For this review, take the finished solid that the model builds, in its own axes (mm). Give positions to 0.01 mm unless a question says otherwise; leave off trailing zeros. Write each loop counter-clockwise with the first axis right and the second up, starting at its lowest first coordinate (ties: lowest second). Pieces come first, ordered by that corner, then holes. Notation, with made-up numbers: (9, 49.5) -> (67, 49.5) arc R12 ccw to (67, 66.5) -> close; hole circle Ø2 at (-12, 33). An arc over 180 degrees is marked (long way). Return JSON: item names as keys, results as strings.
from build123d import *

# Parameters (mm, degrees)
CYLINDER170_R         = 6.5
CYLINDER170_DEPTH     = 10
ARRAY001_COUNT        = 6
ARRAY001_ANGLE        = 170
CYLINDER012_R         = 2.579687
CYLINDER012_DEPTH     = 19.5
ARRAY_COUNT           = 6
ARRAY_ANGLE           = 208
ARRAY_PLACEMENT_ANGLE = 109
CYLINDER052_R         = 47.75
CYLINDER052_DEPTH     = 3
CYLINDER051_R         = 51.25
CYLINDER051_DEPTH     = 3
CYLINDER164_R         = 2.28
CYLINDER164_DEPTH     = 29
CYLINDER163_R         = 2.58
CYLINDER163_DEPTH     = 29
CYLINDER159_R         = 9
CYLINDER159_DEPTH     = 21
CYLINDER165_R         = 4
CYLINDER165_DEPTH     = 10
CYLINDER166_R         = 4
CYLINDER166_DEPTH     = 10
CYLINDER167_R         = 4
CYLINDER167_DEPTH     = 10
CYLINDER168_R         = 4
CYLINDER168_DEPTH     = 10
CYLINDER005_R         = 51
CYLINDER005_DEPTH     = 20
CYLINDER004_R         = 70.0875
CYLINDER004_DEPTH     = 20
BOX_W                 = 193
BOX_H                 = 248
BOX_DEPTH             = 6.2
FILLET_R              = 80


with BuildPart() as array001:
    # Cylinder170 → Cylinder170 (new body)
    with BuildSketch(Plane(origin=(60, 181, 0), x_dir=(1, 0, 0), z_dir=(0, 0, 1))):
        Circle(CYLINDER170_R)
    extrude(amount=CYLINDER170_DEPTH)

    # Array001: Array001 ×6 about axis
    array001_axis = Axis((0, 176, 0), (0, 0, 1))


with BuildPart() as array001_1:
    add(array001.part)
    for i in range(1, ARRAY001_COUNT):
        add(array001.part.rotate(array001_axis, i * ARRAY001_ANGLE / (ARRAY001_COUNT - 1)))


with BuildPart() as array001_2:
    # Array001 placement: moved
    add(array001_1.part.moved(Location((0, -5, 0))))


with BuildPart() as obj1:
    # Cylinder012 → Cylinder012 (new body)
    with BuildSketch(Plane(origin=(36.025, 58.5, -4), x_dir=(1, 0, 0), z_dir=(0, 0, 1))):
        Circle(CYLINDER012_R)
    extrude(amount=CYLINDER012_DEPTH)

    # Array: obj1 ×6 about axis
    array_axis = Axis((0, 0, 0), (0, 0, 1))


with BuildPart() as obj1_1:
    add(obj1.part)
    for i in range(1, ARRAY_COUNT):
        add(obj1.part.rotate(array_axis, i * ARRAY_ANGLE / (ARRAY_COUNT - 1)))


with BuildPart() as obj1_2:
    # Array placement: moved
    add(obj1_1.part.moved(Location((0, 102, 0))).rotate(Axis((0, 102, 0), (0, 0, 1)), ARRAY_PLACEMENT_ANGLE))


with BuildPart() as flange002:
    # Cylinder052 → Cylinder052 (new body)
    with BuildSketch(Plane(origin=(0, 68, 0), x_dir=(1, 0, 0), z_dir=(0, 0, 1))):
        Circle(CYLINDER052_R)
    extrude(amount=CYLINDER052_DEPTH)


with BuildPart() as centeringringgroove:
    # Cylinder051 → Cylinder051 (new body)
    with BuildSketch(Plane(origin=(0, 68, 0), x_dir=(1, 0, 0), z_dir=(0, 0, 1))):
        Circle(CYLINDER051_R)
    extrude(amount=CYLINDER051_DEPTH)

    # Cut001: cut Flange002
    add(flange002.part, mode=Mode.SUBTRACT)


with BuildPart() as centeringringgroove_1:
    # Cut001 placement: moved
    add(centeringringgroove.part.moved(Location((0, 35, 0))))


with BuildPart() as cylinder016:
    # Cylinder164 → Cylinder164 (new body)
    with BuildSketch(Plane(origin=(15, 33, -9), x_dir=(1, 0, 0), z_dir=(0, 0, 1))):
        Circle(CYLINDER164_R)
    extrude(amount=CYLINDER164_DEPTH)


with BuildPart() as cylinder015:
    # Cylinder163 → Cylinder163 (new body)
    with BuildSketch(Plane(origin=(-14.5, 33.7, -7), x_dir=(1, 0, 0), z_dir=(0, 0, 1))):
        Circle(CYLINDER163_R)
    extrude(amount=CYLINDER163_DEPTH)


with BuildPart() as cylinder011:
    # Cylinder159 → Cylinder159 (new body)
    with BuildSketch(Plane(origin=(0, 67, -4), x_dir=(1, 0, 0), z_dir=(0, 0, 1))):
        Circle(CYLINDER159_R)
    extrude(amount=CYLINDER159_DEPTH)


with BuildPart() as cylinder017:
    # Cylinder165 → Cylinder165 (new body)
    with BuildSketch(Plane(origin=(-87, 173, 0), x_dir=(1, 0, 0), z_dir=(0, 0, 1))):
        Circle(CYLINDER165_R)
    extrude(amount=CYLINDER165_DEPTH)


with BuildPart() as cylinder018:
    # Cylinder166 → Cylinder166 (new body)
    with BuildSketch(Plane(origin=(87, 68, 0), x_dir=(1, 0, 0), z_dir=(0, 0, 1))):
        Circle(CYLINDER166_R)
    extrude(amount=CYLINDER166_DEPTH)


with BuildPart() as cylinder019:
    # Cylinder167 → Cylinder167 (new body)
    with BuildSketch(Plane(origin=(-87, 68, 0), x_dir=(1, 0, 0), z_dir=(0, 0, 1))):
        Circle(CYLINDER167_R)
    extrude(amount=CYLINDER167_DEPTH)


with BuildPart() as cylinder020:
    # Cylinder168 → Cylinder168 (new body)
    with BuildSketch(Plane(origin=(87, 173, 0), x_dir=(1, 0, 0), z_dir=(0, 0, 1))):
        Circle(CYLINDER168_R)
    extrude(amount=CYLINDER168_DEPTH)


with BuildPart() as cylinder005:
    # Cylinder005 → Cylinder005 (new body)
    with BuildSketch(Plane(origin=(0, 74, 0), x_dir=(1, 0, 0), z_dir=(0, 0, 1))):
        Circle(CYLINDER005_R)
    extrude(amount=CYLINDER005_DEPTH)


with BuildPart() as fusion001:
    # Cylinder004 → Cylinder004 (new body)
    with BuildSketch(Plane(origin=(0, 149, 0), x_dir=(1, 0, 0), z_dir=(0, 0, 1))):
        Circle(CYLINDER004_R)
    extrude(amount=CYLINDER004_DEPTH)

    # Common: intersect Cylinder005
    add(cylinder005.part, mode=Mode.INTERSECT)


with BuildPart() as fusion001_1:
    # Common placement: moved
    add(fusion001.part.moved(Location((0, 29, 0))))

    # Fusion: union obj1, CenteringRingGroove, Cylinder016, Cylinder015, Cylinder011, Cylinder017, Cylinder018, Cylinder019, Cylinder020
    add(obj1_2.part)
    add(centeringringgroove_1.part)
    add(cylinder016.part)
    add(cylinder015.part)
    add(cylinder011.part)
    add(cylinder017.part)
    add(cylinder018.part)
    add(cylinder019.part)
    add(cylinder020.part)

    # Fusion001: union Array001
    add(array001_2.part)


with BuildPart() as cut021:
    # Box → Box (new body)
    with BuildSketch(Plane(origin=(-96.5, 0, 0), x_dir=(1, 0, 0), z_dir=(0, 0, 1))):
        with Locations((96.5, 124)):
            Rectangle(BOX_W, BOX_H)
    extrude(amount=BOX_DEPTH)

    # Fillet
    fillet_edges = [cut021.edges().sort_by_distance(p)[0] for p in [
        (-96.5, 0, 3.1),
        (-96.5, 248, 3.1),
        (96.5, 0, 3.1),
        (96.5, 248, 3.1),
    ]]
    fillet(fillet_edges, radius=FILLET_R)

    # Cut021: cut Fusion001
    add(fusion001_1.part, mode=Mode.SUBTRACT)


solid = cut021.part
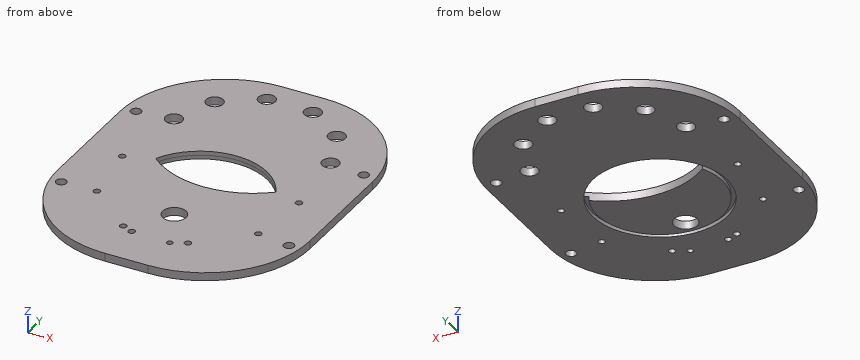
1. Add section A-A, the plane x = 87. State the section outline as (y, z) points, plus the area to 3 significant figures.
Results found:
{"outline": "(42.19, 0) -> (64, 0) -> (64, 6.2) -> (42.19, 6.2) -> close; (72, 0) -> (169, 0) -> (169, 6.2) -> (72, 6.2) -> close; (177, 0) -> (205.81, 0) -> (205.81, 6.2) -> (177, 6.2) -> close", "area": "915 mm²"}
2. Add section D-D, the plane x = -35.5. State the section outline as (y, z) points, plus the area to 3 significant figures.
Results found:
{"outline": "(2.29, 0) -> (66.04, 0) -> (66.04, 3) -> (71.07, 3) -> (71.07, 0) -> (117.57, 0) -> (117.57, 6.2) -> (2.29, 6.2) -> close; (139.62, 3) -> (139.96, 3) -> (139.96, 0) -> (245.71, 0) -> (245.71, 6.2) -> (139.62, 6.2) -> close", "area": "1,360 mm²"}
3. For pin 1 (17 mm diameter, centred on x = 60, y = 176, fed in from -Z); pin 2 (1 mm diameter, centred on x = -32, z = 3, fed in from +Y); pin 3 (1.5 mm diameter, centred on y = 49.5, z = 1.5, fed in from -X), all flat-tipped, find the tip position at first contact; note any pin that passes through.
Results found:
{"pin 1": "stops at z = 0", "pin 2": "stops at y = 246.58", "pin 3": "stops at x = -90.76"}
4. To check wall thickness, follow probe 1 along Y at (x, z) = (-61, 4.5); probe 2 along Y at (x, z) = (87, 3.5); probe 3 along Y at (x, z) = (13, 5). State the ranges of each line that lie inside material, in increasing order.
Results found:
{"probe 1": "y = 13.52 to 66.3, 71.14 to 170.08, 182.91 to 234.48", "probe 2": "y = 42.19 to 64, 72 to 169, 177 to 205.81", "probe 3": "y = 0 to 31.91, 34.09 to 109.13, 152.32 to 224.17, 232.84 to 248"}
5. Add section C-C, the plane y = 103. State the section outline as (x, z) points, plus the area to 3 significant figures.
Results found:
{"outline": "(-96.5, 0) -> (-51.25, 0) -> (-51.25, 3) -> (-47.75, 3) -> (-47.75, 0) -> (47.75, 0) -> (47.75, 3) -> (51.25, 3) -> (51.25, 0) -> (96.5, 0) -> (96.5, 6.2) -> (-96.5, 6.2) -> close", "area": "1,180 mm²"}
6. Add section B-B, the plane y = 143.5. State the section outline as (x, z) points.
Results found:
{"outline": "(-96.5, 0) -> (-31.41, 0) -> (-31.41, 3) -> (-31, 3) -> (-31, 6.2) -> (-96.5, 6.2) -> close; (31, 3) -> (31.41, 3) -> (31.41, 0) -> (96.5, 0) -> (96.5, 6.2) -> (31, 6.2) -> close"}
